Input: part model. Units: mm. Frame: model coordinates. Give positions to 0.01 mm unless a question says otherwise; leave off trailing zeros. Write each loop counter-clockwise with the first axis right and the second up, starting at its lowest first coordinate (ties: lowest second). Pieces come first, ordered by that corner, then holes.
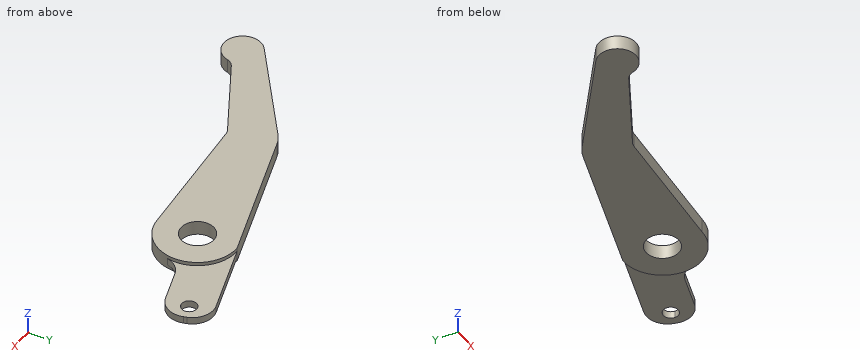
```python
from build123d import *

# Parameters (mm, degrees)
SKETCH1_R           = 14
BOSS_EXTRUDE1_DEPTH = 12
BOSS_EXTRUDE2_DEPTH = 9
FILLET1_R           = 17.78
CUT_EXTRUDE2_START  = -3
CUT_EXTRUDE2_DEPTH  = 3


with BuildPart() as part:
    # Sketch1 → Boss-Extrude1 (new body)
    with BuildSketch(Plane.XY):
        with BuildLine():
            Line((-96.91554928, -1.121955778), (-15.722399936, 58.140946839))
            ThreePointArc((-15.722399936, 58.140946839), (-11.394783315, 60.770107897), (-6.686327841, 62.633223709))
            Line((-6.686327841, 62.633223709), (112.446127039, 98.471593282))
            ThreePointArc((112.446127039, 98.471593282), (145.896391136, 65.021329185), (112.446127039, 31.571065087))
            Line((112.446127039, 31.571065087), (2.176317829, 24.613004518))
            ThreePointArc((2.176317829, 24.613004518), (0.064344939, 24.249840519), (-1.921888512, 23.445356673))
            Line((-1.921888512, 23.445356673), (-67.204247556, -11.552416003))
            ThreePointArc((-67.204247556, -11.552416003), (-70.352621766, -14.199342537), (-72.170382748, -17.889088499))
            ThreePointArc((-72.170382748, -17.889088499), (-96.461185182, -27.094594937), (-96.91554928, -1.121955778))
        make_face()
        with Locations((112.446127039, 65.021329185)):
            Circle(SKETCH1_R, mode=Mode.SUBTRACT)
    extrude(amount=-BOSS_EXTRUDE1_DEPTH)

    # Sketch2 → Boss-Extrude2 (add)
    with BuildSketch(Plane.XY):
        with BuildLine():
            Line((179.335031787, 118.593643911), (112.446127039, 98.471593282))
            ThreePointArc((112.446127039, 98.471593282), (134.765386203, 89.936602382), (145.694919218, 68.687115155))
            Line((145.694919218, 68.687115155), (190.310695767, 82.108786775))
            Line((190.310695767, 82.108786775), (186.652141107, 94.270405821))
            ThreePointArc((186.652141107, 94.270405821), (178.742054254, 98.521938013), (182.993586447, 106.432024866))
            Line((182.993586447, 106.432024866), (179.335031787, 118.593643911))
        make_face()
        with BuildLine():
            Line((191.496650832, 122.252198571), (179.335031787, 118.593643911))
            Line((179.335031787, 118.593643911), (182.993586447, 106.432024866))
            ThreePointArc((182.993586447, 106.432024866), (188.611437978, 105.447214315), (191.172863777, 100.351215343))
            ThreePointArc((191.172863777, 100.351215343), (189.918862749, 96.562641142), (186.652141107, 94.270405821))
            Line((186.652141107, 94.270405821), (190.310695767, 82.108786775))
            Line((190.310695767, 82.108786775), (202.472314812, 85.767341435))
            Line((202.472314812, 85.767341435), (191.496650832, 122.252198571))
        make_face()
    extrude(amount=-BOSS_EXTRUDE2_DEPTH)

    # Fillet1
    fillet1_edges = [part.edges().sort_by_distance(p)[0] for p in [
        (191.496650832, 122.252198571, -4.5),
        (202.472314812, 85.767341435, -4.5),
        (145.694919218, 68.687115155, -4.5),
    ]]
    fillet(fillet1_edges, radius=FILLET1_R)

    # Sketch4 → Cut-Extrude2 (cut)
    with BuildSketch(Plane.XY.offset(CUT_EXTRUDE2_START)):
        with BuildLine():
            Line((174.470384169, 117.130222047), (112.446127039, 98.471593282))
            ThreePointArc((112.446127039, 98.471593282), (138.257160255, 86.298329266), (145.281823298, 58.638757657))
            ThreePointArc((145.281823298, 58.638757657), (149.548777584, 67.172961066), (157.613182204, 72.272461516))
            Line((157.613182204, 72.272461516), (185.446048149, 80.645364911))
            ThreePointArc((185.446048149, 80.645364911), (195.985244574, 89.254027292), (197.350338288, 102.793608099))
            Line((197.350338288, 102.793608099), (196.618627356, 105.225931908))
            ThreePointArc((196.618627356, 105.225931908), (188.009964976, 115.765128333), (174.470384169, 117.130222047))
        make_face()
    extrude(amount=CUT_EXTRUDE2_DEPTH, mode=Mode.SUBTRACT)


solid = part.part
```
Q1. Section B-B, the plane z = -5.5. Give the number of separate pieces and of enclosed holes in the cut face, then the cut area to 3 significant figures.
Q2. Section C-C, the plane y = 10. Return the cut outline in (x, z).
Q3. Material intervals for line 1 along Y through (x, z) = (180, -4.5); line 2 along X through (y, z) = (-18, -5.25); line 3 along Y through (x, z) = (-33, -9), sorted ascending.
Q4. Section D-D, the plane x = -28. Return the cut outline in (y, z), then the cut area to 3 significant figures.
Q5. Pin query (flat end, axial travel): pin 1 (1.5 mm diameter, centred on y = -14.5, z = -2.5, fed in from +X); pin 2 (18 mm diameter, centred on x = 146.5, y = 83, fed in from -Z); pin 3 (4 mm diameter, centred on x = -46, z = -10.5, fed in from +Y); pin 4 (5 mm diameter, centred on x = -30, z = -5.5, fed in from +Y). Return the tip coordinate at first contact, or that it passes through.
Q6. Section A-A, the plane x = 134. Return the cut outline in (y, z).
Solutions:
1. separate pieces: 1
1. enclosed holes: 2
1. area: 13,100 mm2
2. outline: (-81.68, -12) - (-27, -12) - (-27, 0) - (-81.68, 0) - close
3. line 1: y = 79.01 to 96.22, 104.48 to 117.88
3. line 2: x = -102.91 to -72.2
3. line 3: y = 6.78 to 45.53
4. outline: (9.46, -12) - (49.18, -12) - (49.18, 0) - (9.46, 0) - close
4. area: 477 mm2
5. pin 1: stops at x = -69.98
5. pin 2: stops at z = -12
5. pin 3: stops at y = 37.5
5. pin 4: stops at y = 49.54
6. outline: (39.44, -12) - (90.6, -12) - (90.6, -9) - (104.96, -9) - (104.96, -3) - (90.6, -3) - (90.6, 0) - (39.44, 0) - close
